Build history of the part. All positions in model axes, mm. A direction names the side the tool comes from. Coordinates: 2 decimals unless noted, no trailing zeros. Loops run counter-clockwise (first coordinate to the right, second up) from the corner with the lowest first, then second, coordinate; pieces in that order, holes last.
Item 1: Cut at B-B (z = 0.9). Count the separate pieces of the cut face and the enclosed holes in it, and give its area (3 significant figures).
Item 2: Cut at D-D (x = 71). List the corners of the cut face in (y, z) (3 decimals), and give its area (3 significant figures).
Item 3: Flat gauge pins, fed straight in: pin 1 (3 mm diameter, centred on x = 79.375, y = -85.725, fed in from +Z) (3 decimals); pin 2 (0.6 mm diameter, centred on y = -96.5, z = 2.5, fed in from +X) (3 decimals); pin 3 (1 mm diameter, centred on x = 54, z = 1.5, fed in from +Y); pin 4 (1.6 mm diameter, centred on x = 54, z = 2, fed in from -Y). Where does each tip first touch, or does it go through?
Item 4: Cut at C-C (y = 0). List the corners of the cut face in (x, z) (3 decimals).
Item 5: 3-axis set-ups, long thin cutter, end or side, ignore diameter. For faces 4 (the face through (62, -96.139, 2)), 5 (the face through (36, -98.425, 2)): which of +Z, -Z, +X, -X, +Y, -Y reach the whole face in a straight line?
Item 6: Cut at A-A (x = 0). List the corners of the cut face in (y, z) (3 decimals).
Item 7: Mould opens along Y. For faces 1 (the face through (62, -49.911, 2)), 2 (the face through (9.315, -49.586, 1.565)), 3 (the face through (53.435, -57.895, 1.565)) say: released by +Y, released by -Y, zero draft, split by the parting line, or undercut.
Item 8: Drill centre lines: line 1 along Y through (x, z) = (79, 2.7); line 2 along Y through (x, z) = (81.5, 1.75); line 3 along X through (y, z) = (-60.5, 2) (3 decimals). Where is each one in solid material? Low to high.
Autodesk Inventor part; units mm, degrees
ref_plane "YZ Plane" through (0, 0, 0) normal (1, 0, 0) x (0, 1, 0)
ref_plane "XZ Plane" through (0, 0, 0) normal (0, 1, 0) x (-1, 0, 0)
ref_plane "XY Plane" through (0, 0, 0) normal (0, 0, 1) x (1, 0, 0)
sketch "Sketch1" plane through (0, 0, 0) normal (0, 0, 1) x (1, 0, 0)
  arc A0 (8.0581, 5.0787) -> (-8.8609, -3.4943) centre (0, 0) ccw
  line L0 (8.0581, 5.0787) -> (41.275, -47.625)
  line L1 (41.275, -47.625) -> (41.275, -49.911)
  line L2 (41.275, -49.911) -> (85.725, -49.911)
  line L3 (85.725, -49.911) -> (85.725, -96.139)
  line L4 (28.575, -98.425) -> (-8.8609, -3.4943)
  circle A1 centre (0, 0) radius 3.2512
  line L5 (85.725, -96.139) -> (41.275, -96.139)
  line L6 (41.275, -96.139) -> (41.275, -98.425)
  line L7 (41.275, -98.425) -> (28.575, -98.425)
  line L8 (85.725, -73.025) -> (85.7238, -73.025) construction
  circle A2 centre (79.375, -60.325) radius 2.4892
  circle A3 centre (66.675, -60.325) radius 2.4892
  circle A4 centre (79.375, -85.725) radius 2.4892
  circle A5 centre (66.675, -85.725) radius 2.4892
  circle A6 centre (53.975, -60.325) radius 2.4892
  circle A7 centre (53.975, -85.725) radius 2.4892
  line L9 (-9.525, 139.734) -> (-9.525, 40.2644) construction
  line L10 (-53.9331, -9.525) -> (112.0207, -9.525) construction
  dimension "d0" = 19.05
  dimension "d1" = 6.5024
  dimension "d2" = 2.286
  dimension "d3" = 4.9784
  dimension "d6" = 12.7
  dimension "d9" = 25.4
  dimension "d12" = 12.7
  dimension "d13" = 50.8
  dimension "d14" = 6.35
  dimension "d15" = 12.7
  dimension "d16" = 50.8
  dimension "d17" = 12.7
  dimension "d18" = 38.1
extrude "Extrusion1" add sketch "Sketch1" along normal blind 3.175
fillet "Fillet1" radius 3.175 2 edges at (85.725, -49.911, 1.5875) (85.725, -96.139, 1.5875)
fillet "Fillet1" radius 6.35 2 edges at (28.575, -98.425, 1.5875) (41.275, -47.625, 1.5875)
fillet "Fillet1" radius 1.5875 1 edges at (41.275, -98.425, 1.5875)
properties part number "VersaChassis Bumper Support Plate" material "Aluminum 6061"
Filled sheet:
1. separate pieces: 1
1. enclosed holes: 7
1. area: 4,490 mm2
2. outline: (-96.139, 0) - (-49.911, 0) - (-49.911, 3.175) - (-96.139, 3.175) - close
2. area: 147 mm2
3. pin 1: passes through
3. pin 2: stops at x = 41.275
3. pin 3: stops at y = -49.91
3. pin 4: stops at y = -96.14
4. outline: (-9.525, 0) - (-3.251, 0) - (-3.251, 3.175) - (-9.525, 3.175) - close; (3.251, 0) - (11.259, 0) - (11.259, 3.175) - (3.251, 3.175) - close
5. face 4: +Z, -Z, +X, -Y
5. face 5: +Z, -Z, +X, -X, -Y
6. outline: (-25.964, 0) - (-3.251, 0) - (-3.251, 3.175) - (-25.964, 3.175) - close; (3.251, 0) - (9.525, 0) - (9.525, 3.175) - (3.251, 3.175) - close
7. face 1: released by +Y
7. face 2: released by -Y
7. face 3: undercut
8. line 1: y = -96.14 to -88.19, -83.26 to -62.79, -57.86 to -49.91
8. line 2: y = -96.14 to -87.02, -84.43 to -61.62, -59.03 to -49.91
8. line 3: x = 13.619 to 51.492, 56.458 to 64.192, 69.158 to 76.892, 81.858 to 85.725
